Autodesk Inventor part; units mm, degrees
ref_plane "YZ Plane" through (0, 0, 0) normal (1, 0, 0) x (0, 1, 0)
ref_plane "XZ Plane" through (0, 0, 0) normal (0, 1, 0) x (-1, 0, 0)
ref_plane "XY Plane" through (0, 0, 0) normal (0, 0, 1) x (1, 0, 0)
sketch "Sketch1" plane through (0, 0, 0) normal (0, 0, 1) x (1, 0, 0)
  line L0 (-15.9035, 8.2993) -> (24.0965, 8.2993)
  line L1 (24.0965, 8.2993) -> (24.0965, -21.7007)
  line L2 (24.0965, -21.7007) -> (-15.9035, -21.7007)
  line L3 (-15.9035, -21.7007) -> (-15.9035, 8.2993)
  point P0 (0, 0)
  dimension "d0" = 40
  dimension "d1" = 30
extrude "Extrusion1" add sketch "Sketch1" along normal blind 2
sketch "Sketch2" plane through (0, 0, 2) normal (0, 0, 1) x (1, 0, 0)
  line L0 (-15.9035, -21.7007) -> (-15.9035, 8.2993)
  line L1 (24.0965, -21.7007) -> (-15.9035, -21.7007)
  line L2 (-15.9035, -6.7007) -> (4.0965, -6.7007)
  line L3 (4.0965, -6.7007) -> (4.0965, -14.7007)
  line L4 (4.0965, -14.7007) -> (-3.9035, -14.7007)
  line L5 (-3.9035, -14.7007) -> (-3.9035, 1.2993)
  line L6 (-3.9035, 1.2993) -> (12.0965, 1.2993)
  line L7 (12.0965, 1.2993) -> (12.0965, -14.7007)
  circle A0 centre (12.0965, -6.7007) radius 1
  circle A1 centre (12.0965, 1.2993) radius 1
  circle A2 centre (4.0965, 1.2993) radius 1
  circle A3 centre (-3.9035, 1.2993) radius 1
  circle A4 centre (-3.9035, -6.7007) radius 1
  circle A5 centre (-3.9035, -14.7007) radius 1
  circle A6 centre (4.0965, -14.7007) radius 1
  circle A7 centre (12.0965, -14.7007) radius 1
  point P0 (0, 0)
  dimension "d4" = 8
  dimension "d5" = 8
  dimension "d6" = 16
  dimension "d7" = 16
  dimension "d8" = 16
  dimension "d9" = 2
extrude "Extrusion2" cut sketch "Sketch2" against normal blind 2 contours A7 | A0 L7 | L7 A0 | A1 L7 L6 | L6 L7 A1 | A2 L6 | L6 A2 | A3 L6 L5 | L5 L6 A3 | A4 L5 L2 | L2 L5 A4 | L5 A4 L2 | L2 A4 L5 | A6 L4 L3 | L3 L4 A6 | A5 L4 L5 | L5 L4 A5
sketch "Sketch3" plane through (-15.9035, -21.7007, 0) normal (0, -1, 0) x (1, 0, 0)
  line L0 (40, 2) -> (0, 2)
  line L1 (0, 0) -> (0, 2)
  line L2 (40, 0) -> (0, 0)
  line L3 (40, 0) -> (40, 2)
  point P0 (15.9035, 0)
extrude "Extrusion3" add sketch "Sketch3" along normal blind 1
sketch "Sketch4" plane through (-15.9035, 8.2993, 0) normal (0, 1, 0) x (1, 0, 0)
  line L0 (0, -2) -> (40, -2)
  line L1 (40, 0) -> (40, -2)
  line L2 (0, 0) -> (40, 0)
  line L3 (0, 0) -> (0, -2)
  point P0 (15.9035, 0)
extrude "Extrusion4" add sketch "Sketch4" along normal blind 1
sketch "Sketch7" plane through (-15.9035, -22.7007, 0) normal (0, -1, 0) x (1, 0, 0)
  line L0 (40, 0) -> (0, 0)
  line L1 (0, 2) -> (1, 2)
  line L2 (1, 2) -> (1, 0)
  line L3 (1, 0) -> (0, 0)
  line L4 (0, 0) -> (0, 2)
  point P0 (15.9035, 0)
  dimension "d18" = 1
extrude "Extrusion6" cut sketch "Sketch7" against normal blind 50.8
properties part number "base1"
Could you check a few things on this model? Use its own coordinates, in mm. Coordinates: 2 decimals unless noted, no trailing zeros.
1. For P1, Ø2.5, axis at x = -3.9, y = 1.3, coming from the -Z side, with a flat end and sliding along its axis, tell me the tip position at first contact or that it passes through.
2. I need wall thicknesses on L1, parallel to Y at x = 3.5, z = 0.75; L2, parallel to Y at x = -3, z = 0.15. Which ranges of each line are inside material? Lowest first, please.
3. We'd pull the mould along Y, two halves only. Please class faces 1 (the face through (4, -22.701, 1)), 2 (the face through (11.303, 0.691, 1.014)), 3 (the face through (4, -7, 2)): released by +Y, released by -Y, zero draft, split by the parting line, or undercut.
4. Imagine slicing it at A-A (z = 0.35). Give the number of separate pieces and of enclosed holes in the cut face, and give its area (3 significant figures).
Computed values:
1. P1: stops at z = 0
2. L1: y = -22.7 to -15.5, -13.9 to 0.5, 2.1 to 9.3
2. L2: y = -22.7 to -15.13, -14.27 to -7.13, -6.27 to 0.87, 1.73 to 9.3
3. face 1: released by -Y
3. face 2: undercut
3. face 3: zero draft
4. separate pieces: 1
4. enclosed holes: 8
4. area: 1,220 mm2
